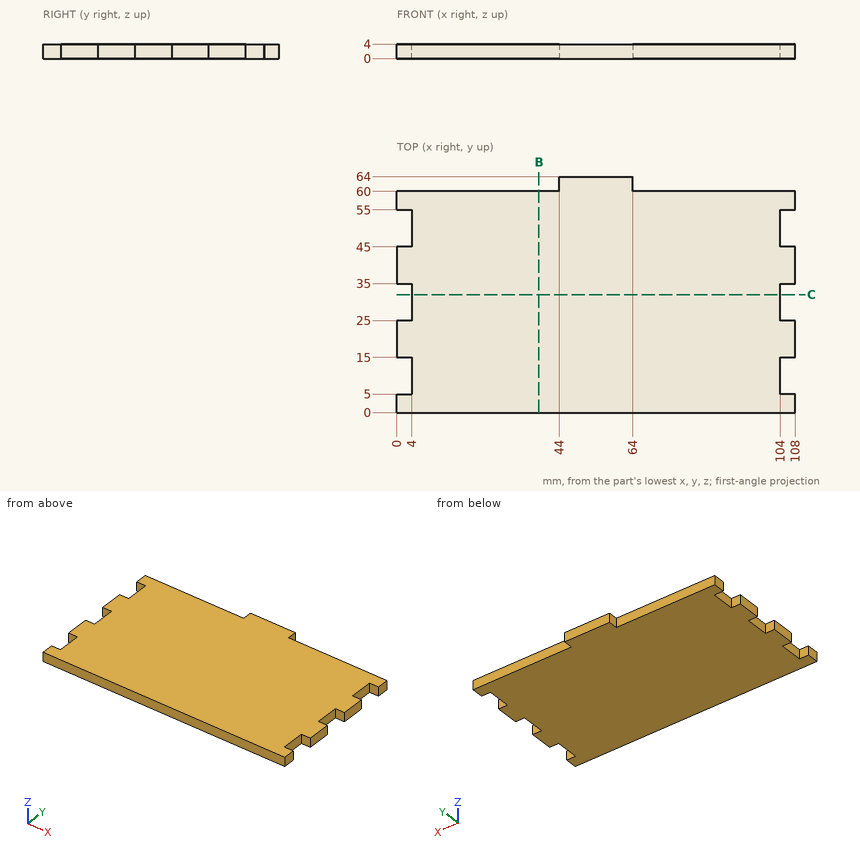
Here's the drawing with two shaded views (mm, measured from the low corner). I have some questions. Give positions to 0.01 mm unless a question says otherwise; leave off trailing zeros. Loops run counter-clockwise (first coordinate to the right, second up) from the corner with the lowest first, then second, coordinate; pieces in that order, holes last. Notation, with made-up numbers: (33, 66.25) -> (91, 66.25) arc R15 ccw to (91, 78.25) -> close; hole circle Ø11 at (-10.75, 37). An arc over 180 degrees is marked (long way). Answer as a JSON object with one key per item and string values. Group by question number.
Item 1: Will these pins go through, and if not, where does the flat tip stop? pin 1 (10 mm diameter, centred on x = 79, y = 11, fed in from -Z); pin 2 (1.2 mm diameter, centred on x = 83.5, z = 1.5, fed in from +Y); pin 3 (1.2 mm diameter, centred on y = 11, z = 3, fed in from -X); pin 4 (2 mm diameter, centred on y = 31, z = 1.5, fed in from +X).
Item 2: I need wall thicknesses on L1, parallel to X at y = 8, z = 0.6; L2, parallel to Y at x = 77, z = 1.7. Which ranges of each line are inside material? Lowest first, please.
Item 3: Imagine slicing it at C-C on y = 32. Write out the boundary of the cut face in (x, z).
Item 4: Imagine slicing it at B-B on x = 38.5. Write out the boundary of the cut face in (y, z).
Answer list:
{
 "1": {"pin 1": "stops at z = 0", "pin 2": "stops at y = 60", "pin 3": "stops at x = 4", "pin 4": "stops at x = 104"},
 "2": {"L1": "x = 4 to 104", "L2": "y = 0 to 60"},
 "3": {"outline": "(4, 0) -> (104, 0) -> (104, 4) -> (4, 4) -> close"},
 "4": {"outline": "(0, 0) -> (60, 0) -> (60, 4) -> (0, 4) -> close"}
}
